The figure shows three views and two pictorial views of one solid part (mm, origin at its lowest corner). Answer the questions. Give positions to 0.01 mm unless a question says otherwise; leave off trailing zeros. Write each loop counter-clockwise with the first axis right and the second up, starting at its lowest first coordinate (ties: lowest second). Pieces come first, ordered by that corner, then holes. Notation, with made-up numbers: (5.25, -7.5) -> (48.25, -7.5) arc R27 ccw to (48.25, 28.5) -> close; hole circle Ø8 at (64, 41). An arc over 180 degrees is marked (long way). Use a Markdown table: item, result.
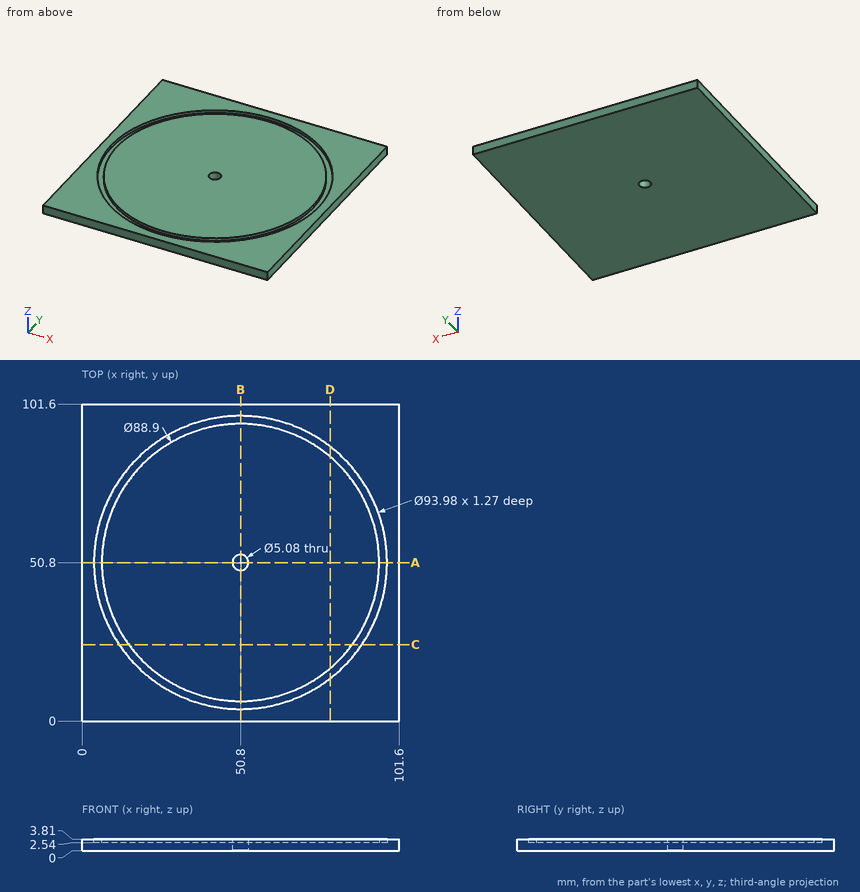
Item 1: This flat-tipped pin is pushed along its axis until it touches: P1, Ø6, axis at x = 50.8, y = 50.8, coming from the -Z side. Where does it stop, or does it pass through?
Return value:
| item | result |
|---|---|
| P1 | z = 0 |
Item 2: Straight lines are drawn through the part: line 1 along Y through (x, z) = (50.8, 3.05); line 2 along Y through (x, z) = (50.8, 1.2); line 3 along Y through (x, z) = (27, 2.7). For each, find the intervals that lie inside material, in ascending order. Write a range as [from, to].
Return value:
| item | result |
|---|---|
| line 1 | [0, 3.81], [6.35, 48.26], [53.34, 95.25], [97.79, 101.6] |
| line 2 | [0, 48.26], [53.34, 101.6] |
| line 3 | [0, 10.28], [13.26, 88.34], [91.32, 101.6] |
Item 3: A cutting plane is placed at D-D (x = 79.5). Give the vertices of the cut face in (y, z), then the cut area to 3 significant figures.
Return value:
| item | result |
|---|---|
| outline | (0, 0) -> (101.6, 0) -> (101.6, 3.81) -> (88.01, 3.81) -> (88.01, 2.54) -> (84.74, 2.54) -> (84.74, 3.81) -> (16.86, 3.81) -> (16.86, 2.54) -> (13.59, 2.54) -> (13.59, 3.81) -> (0, 3.81) -> close |
| area | 379 mm^2 |
Item 4: A cutting plane is placed at C-C (y = 24.5). Give the vertices of the cut face in (x, z).
Return value:
| item | result |
|---|---|
| outline | (0, 0) -> (101.6, 0) -> (101.6, 3.81) -> (89.74, 3.81) -> (89.74, 2.54) -> (86.63, 2.54) -> (86.63, 3.81) -> (14.97, 3.81) -> (14.97, 2.54) -> (11.86, 2.54) -> (11.86, 3.81) -> (0, 3.81) -> close |
Item 5: A cutting plane is placed at A-A (y = 50.8). Give the vertices of the cut face in (x, z).
Return value:
| item | result |
|---|---|
| outline | (0, 0) -> (48.26, 0) -> (48.26, 3.81) -> (6.35, 3.81) -> (6.35, 2.54) -> (3.81, 2.54) -> (3.81, 3.81) -> (0, 3.81) -> close; (53.34, 0) -> (101.6, 0) -> (101.6, 3.81) -> (97.79, 3.81) -> (97.79, 2.54) -> (95.25, 2.54) -> (95.25, 3.81) -> (53.34, 3.81) -> close |
